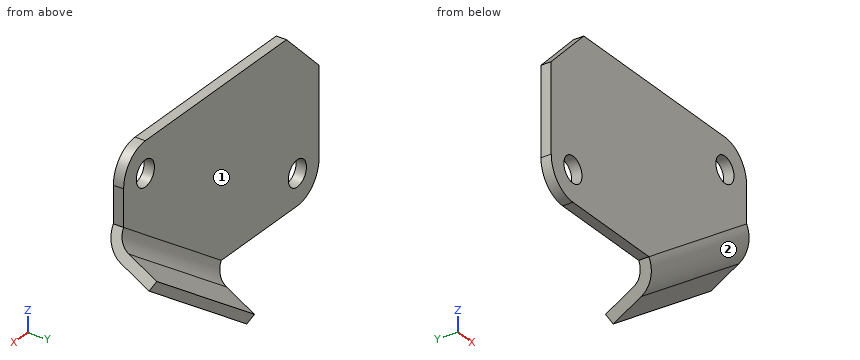
from build123d import *

# Parameters (mm, degrees)
SKETCH1_R           = 5
BOSS_EXTRUDE1_DEPTH = 4
BOSS_EXTRUDE2_DEPTH = 65.921828


with BuildPart() as part:
    # Sketch1 → Boss-Extrude1 (new body)
    with BuildSketch(Plane(origin=(0, 0, 0), x_dir=(1, 0, 0), z_dir=(0, 1, 0))):
        with BuildLine():
            Line((-12, 0), (-12, -34))
            Line((-12, -34), (6, -52))
            Line((6, -52), (84, -52))
            ThreePointArc((84, -52), (92.485281374, -48.485281374), (96, -40))
            Line((96, -40), (96, -25.811207063))
            Line((96, -25.811207063), (42, 12))
            Line((42, 12), (0, 12))
            ThreePointArc((0, 12), (-8.485281374, 8.485281374), (-12, 0))
        make_face()
        Circle(SKETCH1_R, mode=Mode.SUBTRACT)
        with Locations((84, -40)):
            Circle(SKETCH1_R, mode=Mode.SUBTRACT)
    extrude(amount=BOSS_EXTRUDE1_DEPTH)

    # Sketch3 → Boss-Extrude2 (add)
    with BuildSketch(Plane(origin=(76.544267285, 0, 53.59687296), x_dir=(0, -1, 0), z_dir=(0.819152044, 0, 0.573576436))):
        with BuildLine():
            Line((-20.485294843, 50.290733421), (-21.983721217, 46.581998003))
            Line((-21.983721217, 46.581998003), (-9.003147253, 41.337505695))
            ThreePointArc((-9.003147253, 41.337505695), (-5.36769942, 38.393578086), (-4, 33.920034858))
            Line((-4, 33.920034858), (0, 33.920034858))
            ThreePointArc((0, 33.920034858), (-2.051549129, 40.6303497), (-7.504720879, 45.046241113))
            Line((-7.504720879, 45.046241113), (-20.485294843, 50.290733421))
        make_face()
    extrude(amount=-BOSS_EXTRUDE2_DEPTH)


solid = part.part
Verification items for the finished model (mm, model axes). Face numbers are marked on the shaded views. A direction names the side the tool comes from. Coordinates: 2 decimals unless noted, no trailing zeros. Write each loop counter-clockwise with the first axis right and the second up, starting at its lowest first coordinate (ties: lowest second). Pieces come first, ordered by that corner, then holes. Notation, with made-up numbers: (-33, 62.25) - (-11, 62.25) arc R9 ccw to (-11, 74.25) - close; hole circle Ø9 at (3.25, -28). An arc over 180 degrees is marked (long way). Answer as a JSON object with one key per item and string values.
(1) Tool access check on the marked faces 1 and 2. Record the directions out of +Z, -Z, +X, -X, +Y, -Y that give a thin tool (end or side, any length) a straight path to the whole face; none if there is none.
Report:
{"face 1": "+Z, -X, +Y", "face 2": "-Z, +X, -Y"}
(2) Cross-section at B-B on x = 9. Record the cut outline in (y, z), plus the area to 3 significant figures.
Report:
{"outline": "(0, -12) - (4, -12) - (4, 52) - (0, 52) - close", "area": "256 mm^2"}
(3) Cross-section at A-A on z = 37.5. Record the cut outline in (x, y), plus the area to 3 significant figures.
Report:
{"outline": "(-8.5, 0) - (79.67, 0) - (79.67, 4) - (-8.5, 4) - close; (88.33, 0) - (96, 0) - (96, 4) - (88.33, 4) - close", "area": "383 mm^2"}
(4) Gauge pin test, flat ends, axial feed: pin 1 Ø1 at (x, z) = (64.5, 40) entering from +Y; pin 2 Ø4 at (x, y) = (20, 7) entering from -Z; pin 3 Ø3 at (y, z) = (2.5, 36) entering from +X; pin 4 Ø2 at (y, z) = (14.5, 17.5) entering from -X. Record the tip position at first contact, or that the pin passes through.
Report:
{"pin 1": "y = 4", "pin 2": "through", "pin 3": "x = 96", "pin 4": "x = 99.34"}
(5) Thickness scan on line 1 along Y through (x, z) = (7, 32); line 2 along Z through (x, y) = (0, 2.05); line 3 along X through (y, z) = (3.75, -3.5). Record the ranges inside material, lowest first.
Report:
{"line 1": "0 to 4", "line 2": "-12 to -5, 5 to 46", "line 3": "-11.48 to -3.57, 3.57 to 69.33"}
(6) Cross-section at C-C on y = 6.25. Record the cut outline in (x, z).
Report:
{"outline": "(45.19, -16.56) - (48.04, -20.63) - (102.04, 17.18) - (99.19, 21.25) - close"}
